```python
from build123d import *

# Parameters (mm, degrees)
F0_W     = 43
F0_H     = 3
F1_DEPTH = 25
F2_W     = 4.5
F2_H     = 10
F3_DEPTH = 14
F4_R     = 4.99999
F6_DEPTH = 5
F7_W     = 9.8148105666
F7_H     = 8.2614529669
F8_DEPTH = 7


# Not quite as in the source:
# - a fillet or chamfer is up to 0.001 mm smaller than in the source, because OpenCascade refuses the exact size


with BuildPart() as f1:
    # F0 (on Front) → F1 (new body)
    with BuildSketch(Plane.XZ):
        Polygon((0, 52.4), (0, 48.4), (4, 48.4), align=None)
        Polygon((-3, 0), (0, 0), (0, 3), (0, 48.4), (0, 52.4), (-3, 52.4), align=None)
        with Locations((21.5, 1.5)):
            Rectangle(F0_W, F0_H)
        Polygon((43, 3), (43, 0), (46, 0), (46, 47.4), (43, 47.4), align=None)
    extrude(amount=F1_DEPTH)

    # F2 (on face) → F3 (join)
    with BuildSketch(Plane(origin=(0, 0, 0), x_dir=(1, 0, 0), z_dir=(0, 0, -1))):
        with Locations((8.6824605241, 5.0298511051)):
            Rectangle(F2_W, F2_H)
    extrude(amount=F3_DEPTH)

    # F4 (radius 5 in the source; OpenCascade refuses exactly that, so slightly less here)
    f4_edges = [f1.edges().sort_by_distance(p)[0] for p in [
        (8.682461, -10.029851, -14),
        (8.682461, -0.029851, -14),
    ]]
    fillet(f4_edges, radius=F4_R)

    # F5 (on face) → F6 (cut)
    with BuildSketch(Plane(origin=(6.4324605241, 0, 0), x_dir=(0, -1, 0), z_dir=(-1, 0, 0))):
        with BuildLine():
            ThreePointArc((5.0298511051, -7.45), (3.9338580131, -10.0959613868), (6.5798194, -8.9999682949))
            ThreePointArc((6.5798194, -8.9999682949), (6.125844197, -7.9039752029), (5.0298511051, -7.45))
        make_face()
    extrude(amount=-F6_DEPTH, mode=Mode.SUBTRACT)

    # F7 (on face) → F8 (cut)
    with BuildSketch(Plane(origin=(-3, 0, 0), x_dir=(0, -1, 0), z_dir=(-1, 0, 0))):
        with Locations((20.0925947167, 48.2692735165)):
            Rectangle(F7_W, F7_H)
    extrude(amount=-F8_DEPTH, mode=Mode.SUBTRACT)


solid = f1.part
```
Geometry check sheet. Reference: the model listing, model coordinates, mm. A direction names the side the tool comes from. Coordinates: 2 decimals unless noted, no trailing zeros. Order: outer loops, then holes, each group sorted by start corner. A loop starts at its lowest first (then second) coordinate and runs counter-clockwise, first axis right, second up.
Item 1: Depth check by flat-ended pin: pin 1 (1.5 mm diameter, centred on x = 44, y = -9, fed in from +Z); pin 2 (1 mm diameter, centred on x = 25, y = -21, fed in from -Z); pin 3 (3 mm diameter, centred on y = -4, z = -4, fed in from +X); pin 4 (2 mm diameter, centred on y = -16.5, z = -2, fed in from +X). Enter the tip coordinate at first touch or a pass-through.
Item 2: Tool access check on faces 4 (the flat face through (2, -7, 48.4)), 5 (the flat face through (9, -10.03, -4)), 6 (the flat face through (0, -12, 25)), 7 (the flat face through (6.432, -5, -7)), 8 (the flat face through (45, -12, 47.4)). Record the directions out of +Z, -Z, +X, -X, +Y, -Y that give a thin tool (end or side, any length) a straight path to the whole face; none if there is none.
Item 3: Section check D-D (y = -16.25). Enter the section's corners in (x, z).
Item 4: Section check A-A (z = 34.5). Enter the section's corners in (x, y), plus the area to 3 significant figures.
Item 5: Section check B-B (x = 1.5). Enter the section's corners in (y, z).
Item 6: Section check C-C (y = -11). Enter the section's corners in (x, z), plus the area to 3 significant figures.
Item 7: Scan lines: line 1 along X through (y, z) = (-8.75, 39); line 2 along Z through (x, y) = (36, -15.5); line 3 along Z through (x, y) = (-1, -2). Record each from-to range of solid material in increasing order.
Item 8: Mould release check, pull along X, two halves, no side actions. Record for faces 1 (the flat face through (43, -12, 26)), 2 (the flat face through (-3, -12, 27)), 3 (the cylindrical face through (8.7, -8.6, -12.5)): released by +X, released by -X, zero draft, split by the parting line, or undercut.
Check sheet entries:
1. pin 1: stops at z = 47.4
1. pin 2: stops at z = 0
1. pin 3: stops at x = 10.93
1. pin 4: passes through
2. face 4: +X, +Y, -Y
2. face 5: -Z, +X, -X, -Y
2. face 6: +Y, -Y
2. face 7: -Z, -X, +Y, -Y
2. face 8: +Z, +X, +Y, -Y
3. outline: (-3, 0) - (46, 0) - (46, 47.4) - (43, 47.4) - (43, 3) - (0, 3) - (0, 44.14) - (-3, 44.14) - close
4. outline: (-3, -25) - (0, -25) - (0, 0) - (-3, 0) - close; (43, -25) - (46, -25) - (46, 0) - (43, 0) - close
4. area: 150 mm2
5. outline: (-25, 0) - (0, 0) - (0, 3) - (-25, 3) - close; (-15.19, 48.4) - (0, 48.4) - (0, 50.9) - (-15.19, 50.9) - close
6. outline: (-3, 0) - (46, 0) - (46, 47.4) - (43, 47.4) - (43, 3) - (0, 3) - (0, 48.4) - (4, 48.4) - (0, 52.4) - (-3, 52.4) - close
6. area: 436 mm2
7. line 1: x = -3 to 0, 43 to 46
7. line 2: z = 0 to 3
7. line 3: z = 0 to 52.4
8. face 1: undercut
8. face 2: released by -X
8. face 3: zero draft
